Autodesk Inventor part; units mm, degrees
ref_plane "YZ Plane" through (0, 0, 0) normal (1, 0, 0) x (0, 1, 0)
ref_plane "XZ Plane" through (0, 0, 0) normal (0, 1, 0) x (-1, 0, 0)
ref_plane "XY Plane" through (0, 0, 0) normal (0, 0, 1) x (1, 0, 0)
sketch "Esquisse1" plane through (0, 0, 0) normal (0, 0, 1) x (1, 0, 0)
  line L0 (-155, -100) -> (155, -100)
  line L1 (175, -80) -> (175, 80)
  line L2 (155, 100) -> (-155, 100)
  line L3 (-175, 80) -> (-175, -80)
  line L4 (-175, -100) -> (175, 100) construction
  line L5 (175, -100) -> (-175, 100) construction
  line L6 (-155, 100) -> (-155, 80)
  line L7 (-155, 80) -> (-175, 80)
  line L8 (155, 100) -> (155, 80)
  line L9 (155, 80) -> (175, 80)
  line L10 (155, -100) -> (155, -80)
  line L11 (155, -80) -> (175, -80)
  line L12 (-155, -100) -> (-155, -80)
  line L13 (-155, -80) -> (-175, -80)
  circle A0 centre (-141, 90) radius 1.85
  circle A1 centre (-165, 66) radius 1.85
  circle A2 centre (-165, -66) radius 1.85
  circle A3 centre (-141, -90) radius 1.85
  circle A4 centre (141, 90) radius 1.85
  circle A5 centre (165, 66) radius 1.85
  circle A6 centre (165, -66) radius 1.85
  circle A7 centre (141, -90) radius 1.85
  point P0 (0, 0)
  dimension "d43" = 350
  dimension "d44" = 200
  dimension "d45" = 20
  dimension "d46" = 20
  dimension "d47" = 20
  dimension "d48" = 20
  dimension "d49" = 20
  dimension "d50" = 20
  dimension "d51" = 20
  dimension "d52" = 20
  dimension "d53" = 3.7
  dimension "d54" = 3.7
  dimension "d55" = 3.7
  dimension "d56" = 3.7
  dimension "d57" = 3.7
  dimension "d58" = 3.7
  dimension "d59" = 3.7
  dimension "d60" = 3.7
  dimension "d61" = 10
  dimension "d62" = 10
  dimension "d63" = 10
  dimension "d64" = 10
  dimension "d65" = 10
  dimension "d66" = 10
  dimension "d67" = 10
  dimension "d68" = 10
  dimension "d69" = 14
  dimension "d70" = 14
  dimension "d71" = 14
  dimension "d72" = 14
  dimension "d73" = 14
  dimension "d74" = 14
  dimension "d136" = 14
  dimension "d137" = 14
extrude "Extrusion2" add sketch "Esquisse1" along normal blind 6
sketch "Esquisse3" plane through (0, 0, 6) normal (0, 0, 1) x (1, 0, 0)
  line L0 (175, -80) -> (175, 80)
  line L1 (175, -25) -> (175, 25)
  line L2 (175, 25) -> (130, 25)
  line L3 (130, 25) -> (130, -25)
  line L4 (130, -25) -> (175, -25)
  line L5 (155, 100) -> (-155, 100)
  line L6 (-175, -80) -> (-175, 80)
  line L7 (-175, -25) -> (-175, 25)
  line L8 (-175, 25) -> (-130, 25)
  line L9 (-130, 25) -> (-130, -25)
  line L10 (-130, -25) -> (-175, -25)
  point P0 (0, 0)
  dimension "d77" = 45
  dimension "d78" = 50
  dimension "d79" = 75
  dimension "d80" = 50
  dimension "d81" = 45
extrude "Extrusion3" cut sketch "Esquisse3" against normal blind 6
sketch "Esquisse4" plane through (0, 0, 6) normal (0, 0, 1) x (1, 0, 0)
  circle A0 centre (-89.5, 10) radius 3
  circle A1 centre (-89.5, -10) radius 3
  circle A2 centre (89.5, 10) radius 3
  circle A3 centre (89.5, -10) radius 3
  line L0 (-175, 80) -> (-175, 25)
  line L1 (-175, -25) -> (-175, -80)
  line L2 (175, 25) -> (175, 80)
  line L3 (175, -80) -> (175, -25)
  line L4 (155, 100) -> (-155, 100)
  line L5 (-155, -100) -> (155, -100)
  point P0 (0, 0)
  dimension "d84" = 6
  dimension "d85" = 6
  dimension "d86" = 6
  dimension "d87" = 6
  dimension "d88" = 85.5
  dimension "d89" = 85.5
  dimension "d90" = 85.5
  dimension "d91" = 85.5
  dimension "d92" = 90
  dimension "d93" = 90
  dimension "d94" = 90
  dimension "d95" = 90
hole "Perçage2" at (-89.5, 10, 6) at (-89.5, -10, 6) at (89.5, 10, 6) at (89.5, -10, 6) direction (0, 0, -1) diameter 6 depth 8 tip angle 118
sketch "Esquisse5" plane through (0, 0, 6) normal (0, 0, 1) x (1, 0, 0)
  line L0 (-81.5, -42.5) -> (-71.5, -42.5)
  line L1 (-71.5, -42.5) -> (-71.5, 42.5)
  line L2 (-71.5, 42.5) -> (-81.5, 42.5)
  line L3 (-81.5, 42.5) -> (-81.5, -42.5)
  line L4 (-81.5, -42.5) -> (-71.5, 42.5) construction
  line L5 (-71.5, -42.5) -> (-81.5, 42.5) construction
  line L6 (-175, -25) -> (-175, -80)
  line L7 (71.5, -42.5) -> (81.5, -42.5)
  line L8 (81.5, -42.5) -> (81.5, 42.5)
  line L9 (81.5, 42.5) -> (71.5, 42.5)
  line L10 (71.5, 42.5) -> (71.5, -42.5)
  line L11 (71.5, -42.5) -> (81.5, 42.5) construction
  line L12 (81.5, -42.5) -> (71.5, 42.5) construction
  line L13 (130, 25) -> (130, -25)
  line L14 (175, -80) -> (175, -25)
  line L15 (-155, -100) -> (155, -100)
  point P0 (0, 0)
  point P1 (-76.5, 0)
  point P2 (76.5, 0)
  dimension "d103" = 10
  dimension "d104" = 85
  dimension "d107" = 10
  dimension "d108" = 85
  dimension "d111" = 100
  dimension "d112" = 100
  dimension "d134" = 93.5
  dimension "d135" = 93.5
extrude "Extrusion4" cut sketch "Esquisse5" against normal blind 6
sketch "Esquisse6" plane through (0, 0, 6) normal (0, 0, 1) x (1, 0, 0)
  circle A0 centre (-65, 20) radius 2.5
  circle A1 centre (-65, -20) radius 2.5
  circle A2 centre (65, 20) radius 2.5
  circle A3 centre (65, -20) radius 2.5
  line L0 (175, 25) -> (175, 80)
  line L1 (175, -80) -> (175, -25)
  line L2 (-175, 80) -> (-175, 25)
  line L3 (-175, -25) -> (-175, -80)
  line L4 (155, 100) -> (-155, 100)
  line L5 (-155, -100) -> (155, -100)
  point P0 (0, 0)
  dimension "d115" = 5
  dimension "d116" = 5
  dimension "d117" = 5
  dimension "d118" = 5
  dimension "d119" = 110
  dimension "d120" = 110
  dimension "d121" = 110
  dimension "d122" = 110
  dimension "d123" = 80
  dimension "d124" = 80
  dimension "d125" = 80
  dimension "d126" = 80
hole "Perçage3" at (-65, 20, 6) at (-65, -20, 6) at (65, 20, 6) at (65, -20, 6) direction (0, 0, -1) diameter 5 depth 8 tip angle 118
equation "\"d45\" = d51"
equation "\"d46\" = d51"
equation "\"d47\" = d52"
equation "\"d48\" = d51"
equation "\"d49\" = d52"
equation "\"d50\" = d52"
equation "\"d52\" = d51"
equation "\"d54\" = d53"
equation "\"d55\" = d53"
equation "\"d56\" = d53"
equation "\"d57\" = d53"
equation "\"d58\" = d53"
equation "\"d59\" = d53"
equation "\"d60\" = d53"
equation "\"d61\" = d62"
equation "\"d63\" = d62"
equation "\"d64\" = d62"
equation "\"d65\" = d62"
equation "\"d66\" = d62"
equation "\"d67\" = d62"
equation "\"d68\" = d62"
equation "\"d70\" = d69"
equation "\"d71\" = d69"
equation "\"d72\" = d69"
equation "\"d73\" = d69"
equation "\"d74\" = d69"
equation "\"d136\" = d74"
equation "\"d137\" = d69"
equation "\"d85\" = d84"
equation "\"d86\" = d84"
equation "\"d87\" = d84"
equation "\"d89\" = d88"
equation "\"d90\" = d88"
equation "\"d91\" = d88"
equation "\"d93\" = d92"
equation "\"d94\" = d92"
equation "\"d95\" = d93"
properties part number "base" material "Bois (cerisier)"
The listing builds one solid part. Answer for the finished solid, in the listing's coordinates (mm). Give positions to 0.01 mm unless a question says otherwise; leave off trailing zeros. Order: outer loops, then holes, each group sorted by start corner. A loop starts at its lowest first (then second) coordinate and runs counter-clockwise, first axis right, second up. Notation, with made-up numbers: (74.5, 68) -> (90.5, 68) arc R17 ccw to (90.5, 90) -> close; hole circle Ø6 at (26, 20). An arc over 180 degrees is marked (long way). Answer as CSV lines item,"result". Start each with the question number.
Q1. Find the intervals of material crossed by L1, parallel to X at y = -10, z = 4.2; L2, parallel to Y at x = 141, z = 3.85; L3, parallel to Y at x = -89.5, z = 1.7, in increasing order.
Q2. Given pin 1 (3 mm diameter, centred on y = -11.5, z = 4, fed in from -X); pin 2 (1.8 mm diameter, centred on y = -4.5, z = 2, fed in from +X); pin 3 (3 mm diameter, centred on x = -166.5, z = 3.5, fed in from +Y), each flat-ended and moving along its own axis, determine where each tip first touches the part or whether it passes through.
Q3. A cutting plane is placed at B-B (z = 2.5). Count the separate pieces of the cut face and the enclosed holes in it, then the cut area to 3 significant figures.
Q4. A cutting plane is placed at A-A (y = -38.5). Determine the outline of the cut face in (x, z).
Results found:
1,L1,"-130 to -92.5, -86.5 to -81.5, -71.5 to 71.5, 81.5 to 86.5, 92.5 to 130"
1,L2,"-100 to -91.85, -88.15 to -25, 25 to 88.15, 91.85 to 100"
1,L3,"-100 to -13, -7 to 7, 13 to 100"
2,pin 1,"x = -130"
2,pin 2,"x = 130"
2,pin 3,"y = 80"
3,separate pieces,"1"
3,enclosed holes,"18"
3,area,"61,900 mm2"
4,outline,"(-175, 0) -> (-81.5, 0) -> (-81.5, 6) -> (-175, 6) -> close; (-71.5, 0) -> (71.5, 0) -> (71.5, 6) -> (-71.5, 6) -> close; (81.5, 0) -> (175, 0) -> (175, 6) -> (81.5, 6) -> close"
